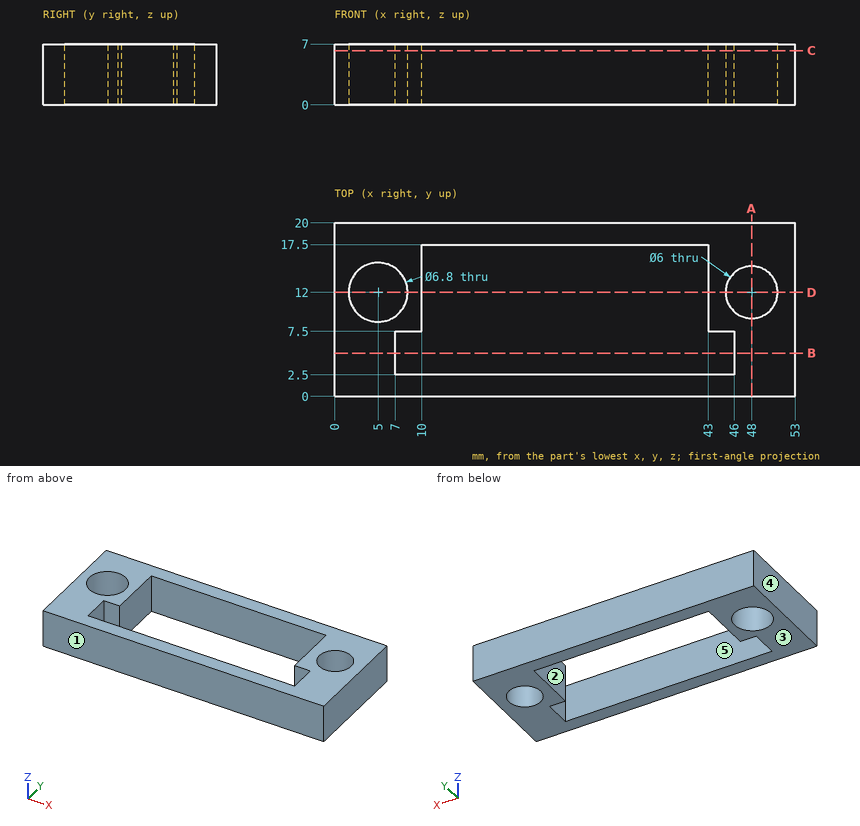
Verification items for this drawing (mm, ordinates from the low corner). A direction names the side the tool comes from. Give positions to 0.01 mm unless a question says otherwise; leave off trailing zeros. Write each loop counter-clockwise with the first axis right and the second up, starting at its lowest first coordinate (ties: lowest second). Pieces come first, ordered by that corner, then holes.
1) Release check for a two-part mould opening along X. For the marked faces 3, 4 and 5 record: pulls with the +X half, pulls with the -X half, needs draft (parallel to the pull), parting line crosses it, or undercut.
2) Section check C-C, the plane z = 6.25. Record the boundary of the cut face in (x, y).
3) Section check A-A, the plane x = 48. Record the boundary of the cut face in (y, z), and give its area (3 significant figures).
4) Gauge pin test, flat end, axial feed: pin 1 (6 mm diameter, centred on x = 5, y = 12, fed in from +Z). Record the tip position at first contact, or that the pin passes through.
5) Access from +Z, -Z, +X, -X, +Y, -Y to the whole of each face (thin tool, end or side, straight path). Record for the marked faces 1 and 2.
6) Material ranges on L1, parallel to X at y = 4, z = 1.75; L2, parallel to Y at x = 5, z = 4.75; L3, parallel to Y at x = 29, z = 4.5, recorded low to high.
7) Section check B-B, the plane y = 5. Record the boundary of the cut face in (x, z), and give its area (3 significant figures).
8) Section check D-D, the plane y = 12. Record the boundary of the cut face in (x, z), and give its area (3 significant figures).
Computed:
1. face 3: needs draft
1. face 4: pulls with the -X half
1. face 5: undercut
2. outline: (0, 0) - (53, 0) - (53, 20) - (0, 20) - close; hole circle Ø6.8 at (5, 12); hole (7, 2.5) - (46, 2.5) - (46, 7.5) - (43, 7.5) - (43, 17.5) - (10, 17.5) - (10, 7.5) - (7, 7.5) - close; hole circle Ø6 at (48, 12)
3. outline: (0, 0) - (9, 0) - (9, 7) - (0, 7) - close; (15, 0) - (20, 0) - (20, 7) - (15, 7) - close
3. area: 98.0 mm2
4. pin 1: passes through
5. face 1: +Z, -Z, +X, -X, -Y
5. face 2: +Z, -Z
6. L1: x = 0 to 7, 46 to 53
6. L2: y = 0 to 8.6, 15.4 to 20
6. L3: y = 0 to 2.5, 17.5 to 20
7. outline: (0, 0) - (7, 0) - (7, 7) - (0, 7) - close; (46, 0) - (53, 0) - (53, 7) - (46, 7) - close
7. area: 98.0 mm2
8. outline: (0, 0) - (1.6, 0) - (1.6, 7) - (0, 7) - close; (8.4, 0) - (10, 0) - (10, 7) - (8.4, 7) - close; (43, 0) - (45, 0) - (45, 7) - (43, 7) - close; (51, 0) - (53, 0) - (53, 7) - (51, 7) - close
8. area: 50.4 mm2
